Check sheet for the modelled part. Datum: model origin and axes. Units: mm. Coordinates: 2 decimals unless noted, no trailing zeros. Order: outer loops, then holes, each group sorted by start corner. A loop starts at its lowest first (then second) coordinate and runs counter-clockwise, first axis right, second up.
from build123d import *

# Parameters (mm, degrees)
SKETCH1_R           = 18
BOSS_EXTRUDE1_DEPTH = 75


with BuildPart() as part:
    # Sketch1 → Boss-Extrude1 (new body)
    with BuildSketch(Plane(origin=(0, 0, 0), x_dir=(1, 0, 0), z_dir=(0, 1, 0))):
        Circle(SKETCH1_R)
        with BuildLine():
            Line((-2, 11.832159566), (-2, 12.832159566))
            Line((-2, 12.832159566), (2, 12.832159566))
            Line((2, 12.832159566), (2, 11.832159566))
            ThreePointArc((2, 11.832159566), (9.16515139, 7.745966692), (12, 0))
            ThreePointArc((12, 0), (-7.745966692, -9.16515139), (-2, 11.832159566))
        make_face(mode=Mode.SUBTRACT)
    extrude(amount=BOSS_EXTRUDE1_DEPTH)


solid = part.part
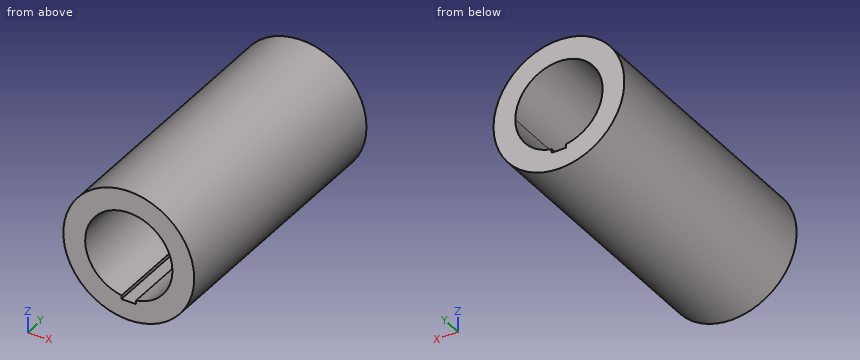
(1) Go/stop test with flat-tipped pins: P1, Ø3, axis at x = 0, y = 38, coming from the +Z side; P2, Ø1.5, axis at x = -6.5, y = 12, coming from the +Z side; P3, Ø10, axis at y = 45, z = -9.5, coming from the -X side. Record where each tip stops, or that it passes through.
Filled in:
P1: stops at z = 18
P2: stops at z = 17.06
P3: stops at x = -17.43
(2) Cross-section at D-D (z = -16). Enter the section's corners in (x, y), and give its area (3 significant figures).
Filled in:
outline: (-8.25, 0) - (8.25, 0) - (8.25, 75) - (-8.25, 75) - close
area: 1,240 mm2
(3) Thickness scan on probe 1 along X at (y, z) = (21.5, 0); probe 2 along Z at (x, y) = (0, 59); probe 3 along X at (y, z) = (41, 3.5). Record the ranges inside material, lowest first.
Filled in:
probe 1: x = -18 to -12, 12 to 18
probe 2: z = -18 to -12.83, 12 to 18
probe 3: x = -17.66 to -11.48, 11.48 to 17.66
(4) Cross-section at C-C (y = 53). Enter the section's corners in (x, z).
Filled in:
outline: circle Ø36 at (0, 0); hole (-2, -12.83) - (2, -12.83) - (2, -11.83) arc R12 ccw (long way) to (-2, -11.83) - close
(5) Cross-section at B-B (z = 4). Enter the section's corners in (x, y), and give its area (3 significant figures).
Filled in:
outline: (-17.55, 0) - (-11.31, 0) - (-11.31, 75) - (-17.55, 75) - close; (11.31, 0) - (17.55, 0) - (17.55, 75) - (11.31, 75) - close
area: 935 mm2
(6) Cross-section at A-A (x = 0). Enter the section's corners in (y, z), and give its area (3 significant figures).
Filled in:
outline: (0, -18) - (75, -18) - (75, -12.83) - (0, -12.83) - close; (0, 12) - (75, 12) - (75, 18) - (0, 18) - close
area: 838 mm2
